Source: CAD feature listing. Evaluate the final solid. Frame: model axes, mm. Face numbers are marked on the shaded views. A direction names the side the tool comes from. Round coordinates to 2 decimals unless told otherwise and drop trailing zeros. Order: outer loops, then holes, each group sorted by start corner. A loop starts at its lowest first (then second) coordinate and runs counter-clockwise, first axis right, second up. Notation, with made-up numbers: M 41.25,-36 L 58.25,-36 A37 cw 58.25,0 Z; hole C 1.5,75 d7. An arc over 180 degrees is marked long. Answer in a Markdown table with one row per item. Add a question column.
```python
from build123d import *

# Parameters (mm, degrees)
SKETCH1_R                = 1.825
BOSS_EXTRUDE1_DEPTH      = 0.75
SKETCH1_4_W              = 5.25
SKETCH1_4_H              = 11
BOSS_EXTRUDE2_DEPTH      = 4
BOSS_EXTRUDE2_DEPTH_BACK = 0.9
SKETCH2_W                = 4.3
SKETCH2_H                = 9.5
BOSS_EXTRUDE3_DEPTH      = 10.1
SKETCH3_R                = 1.1
BOSS_EXTRUDE4_DEPTH      = 1.2
CUT_EXTRUDE1_DEPTH       = 0.4


with BuildPart() as part:
    # Sketch1 → Boss-Extrude1 (new body, symmetric)
    with BuildSketch(Plane(origin=(0, 0, 0), x_dir=(1, 0, 0), z_dir=(0, 1, 0))):
        Polygon((-4.55, 17.7), (-4.55, 12.7), (4.55, 12.7), (4.55, 17.7), (7.45, 17.7), (7.45, -17.7), (-7.45, -17.7), (-7.45, 17.7), align=None)
        with Locations((0, -9.055)):
            Circle(SKETCH1_R, mode=Mode.SUBTRACT)
    extrude(amount=BOSS_EXTRUDE1_DEPTH, both=True)

    # Sketch1_4 → Boss-Extrude2 (add, two sides)
    with BuildSketch(Plane(origin=(0, 0, 0), x_dir=(1, 0, 0), z_dir=(0, 1, 0))) as boss_extrude2_sk:
        with Locations((0, 18.2)):
            Rectangle(SKETCH1_4_W, SKETCH1_4_H)
    extrude(amount=BOSS_EXTRUDE2_DEPTH)
    extrude(boss_extrude2_sk.sketch, amount=-BOSS_EXTRUDE2_DEPTH_BACK)

    # Sketch2 → Boss-Extrude3 (add)
    with BuildSketch(Plane(origin=(0, 0.75, 0), x_dir=(1, 0, 0), z_dir=(0, 1, 0))):
        with Locations((-4.3, -0.45)):
            Rectangle(SKETCH2_W, SKETCH2_H)
    extrude(amount=BOSS_EXTRUDE3_DEPTH)

    # Sketch3 → Boss-Extrude4 (add)
    with BuildSketch(Plane(origin=(0, 10.85, 0), x_dir=(1, 0, 0), z_dir=(0, 1, 0))):
        with Locations((-5.35, -4.1)):
            Circle(SKETCH3_R)
    extrude(amount=BOSS_EXTRUDE4_DEPTH)

    # Sketch4 → Cut-Extrude1 (cut)
    with BuildSketch(Plane(origin=(0, 12.05, 0), x_dir=(1, 0, 0), z_dir=(0, 1, 0))):
        with BuildLine():
            Line((-5.15, -3.018334617), (-5.15, -5.181665383))
            ThreePointArc((-5.15, -5.181665383), (-5.35, -5.2), (-5.55, -5.181665383))
            Line((-5.55, -5.181665383), (-5.55, -3.018334617))
            ThreePointArc((-5.55, -3.018334617), (-5.35, -3), (-5.15, -3.018334617))
        make_face()
    extrude(amount=-CUT_EXTRUDE1_DEPTH, mode=Mode.SUBTRACT)


solid = part.part
```
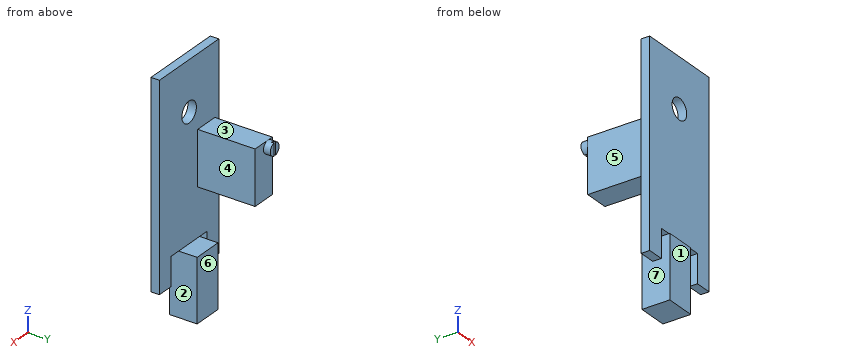
(1) Pin query (flat end, axial travel): pin 1 (1.3 mm diameter, centred on x = -5, z = -0.5, fed in from +Y); pin 2 (1 mm diameter, centred on x = -0.5, y = 2, fed in from +Z); pin 3 (3 mm diameter, centred on x = -3.5, z = -11, fed in from -Y); pin 4 (1.5 mm diameter, centred on y = 1, z = -16, fed in from +X). Return the tip coordinate at first contact, or that it passes through.
(2) Cut plane A-A (x = 0). Return loops of the section in (y, z), and give its area (3 significant figures).
(3) Cut plane B-B (y = 1.75). Return loops of the section in (x, z) (3 decimals).
(4) Line query: line 1 (Z direction, x = 0, y = -0.25); line 2 (Y direction, x = -2.5, z = -8.5); line 3 (Z direction, x = -2.75, y = 2.25). Output: solid intervals per line, ascending. Write a range as from..to.
(5) Cut plane C-C (z = 1). Return loops of the section in (x, y).
(6) Cut plane D-D (x = 5.5). Return loops of the section in (y, z).
(7) Draft query along X for the marked faces 5, 6 and 7. Return one class per face: +X half, -X half, draft (parallel to the pull), parting line (faces both ways), or undercut.
(8) Access query for the marked faces 1, 2, 3 and 4. Directions: +Z, -Z, +X, -X, +Y, -Y. A direction counts if a zero-diameter tool reaches every point of the face in a straight line with its end or side. Return the directions, or none.
Answer list:
| question | item | result |
|---|---|---|
| 1 | pin 1 | y = 10.85 |
| 1 | pin 2 | z = -12.7 |
| 1 | pin 3 | y = -0.75 |
| 1 | pin 4 | x = 7.45 |
| 2 | outline | M -0.9,-23.7 L 4,-23.7 L 4,-12.7 L 0.75,-12.7 L 0.75,7.23 L -0.75,7.23 L -0.75,-12.7 L -0.9,-12.7 Z; M -0.75,10.88 L 0.75,10.88 L 0.75,17.7 L -0.75,17.7 Z |
| 2 | area | 94.0 mm² |
| 3 | outline | M -6.45,-4.3 L -2.15,-4.3 L -2.15,5.2 L -6.45,5.2 Z; M -2.625,-23.7 L 2.625,-23.7 L 2.625,-12.7 L -2.625,-12.7 Z |
| 4 | line 1 | -23.7..7.23, 10.88..17.7 |
| 4 | line 2 | -0.75..0.75 |
| 4 | line 3 | -4.3..5.2 |
| 5 | outline | M -7.45,-0.75 L 7.45,-0.75 L 7.45,0.75 L -2.15,0.75 L -2.15,10.85 L -6.45,10.85 L -6.45,0.75 L -7.45,0.75 Z |
| 6 | outline | M -0.75,-17.7 L 0.75,-17.7 L 0.75,17.7 L -0.75,17.7 Z |
| 7 | face 5 | -X half |
| 7 | face 6 | draft |
| 7 | face 7 | undercut |
| 8 | face 1 | +Z, -Z, +X, -X, -Y |
| 8 | face 2 | -Z, +Y, -Y |
| 8 | face 3 | +Z, +X, -X, +Y |
| 8 | face 4 | +Z, +X, +Y |
